Can you work these out from the model? Positions are in its coordinate system, mm. A direction names the side the tool comes from. Give positions to 0.01 mm unless a question says otherwise; leave off trailing zeros. Order: outer loops, then holes, each group sorted by start corner. A loop starts at its lowest first (then second) coordinate and runs counter-clockwise, first axis right, second up. Notation, with made-up numbers: (12, 44.5) - (39, 44.5) arc R19 cw to (39, 61.5) - close; hole circle Ø2 at (-0.5, 67). An arc over 180 degrees is marked (long way). Answer as a JSON object with one key per item and string values.
```python
from build123d import *

# Parameters (mm, degrees)
EXTRUDE_2_DEPTH = 5


with BuildPart() as part:
    # 草图1 → 凸台-拉伸2 (new body)
    with BuildSketch(Plane(origin=(0, 0, 0), x_dir=(1, 0, 0), z_dir=(0, 1, 0))):
        with BuildLine():
            Line((-5, 0), (7, 0))
            ThreePointArc((7, 0), (9.121320344, 0.878679656), (10, 3))
            Line((10, 3), (10, 6))
            ThreePointArc((10, 6), (10.878679656, 8.121320344), (13, 9))
            Line((13, 9), (177, 9))
            ThreePointArc((177, 9), (179.121320344, 8.121320344), (180, 6))
            Line((180, 6), (180, 3))
            ThreePointArc((180, 3), (180.878679656, 0.878679656), (183, 0))
            Line((183, 0), (195, 0))
            Line((195, 0), (195, 10))
            Line((195, 10), (190, 10))
            Line((190, 10), (190, 15))
            Line((190, 15), (170, 15))
            Line((170, 15), (170, 20))
            Line((170, 20), (160, 20))
            Line((160, 20), (160, 15))
            Line((160, 15), (105, 15))
            Line((105, 15), (105, 20))
            Line((105, 20), (85, 20))
            Line((85, 20), (85, 15))
            Line((85, 15), (30, 15))
            Line((30, 15), (30, 20))
            Line((30, 20), (20, 20))
            Line((20, 20), (20, 15))
            Line((20, 15), (0, 15))
            Line((0, 15), (0, 10))
            Line((0, 10), (-5, 10))
            Line((-5, 10), (-5, 15))
            Line((-5, 15), (-35, 15))
            Line((-35, 15), (-35, 10))
            Line((-35, 10), (-40, 10))
            Line((-40, 10), (-40, 0))
            Line((-40, 0), (-5, 0))
        make_face()
    extrude(amount=EXTRUDE_2_DEPTH)


solid = part.part
```
Q1. If we section it at C-C, the plane x = 124.5: Please give me the cut outline in (y, z), then the cut area to 3 significant figures.
Recorded:
{"outline": "(0, -15) - (5, -15) - (5, -9) - (0, -9) - close", "area": "30.0 mm^2"}
Q2. I need wall thicknesses on L1, parallel to X at y = 3.75, z = -15.5; L2, parallel to X at y = 1.3, z = -3.75; L3, parallel to X at y = 2.65, z = -14.75. Which ranges of each line are inside material? Lowest first, please.
Recorded:
{"L1": "x = 20 to 30, 85 to 105, 160 to 170", "L2": "x = -40 to 10, 180 to 195", "L3": "x = -35 to -5, 0 to 190"}
Q3. If we section it at A-A, the plane z = -17.75: Please give me the cut outline in (x, y), then the cut area to 3 significant figures.
Recorded:
{"outline": "(20, 0) - (30, 0) - (30, 5) - (20, 5) - close; (85, 0) - (105, 0) - (105, 5) - (85, 5) - close; (160, 0) - (170, 0) - (170, 5) - (160, 5) - close", "area": "200 mm^2"}
Q4. I'm going to push flat-ended pins straight in: pin 1 Ø1.5 at (x, y) = (175, 3.5) entering from -Z; pin 2 Ø2.5 at (y, z) = (2, -17) entering from -X; pin 3 Ø1.5 at (x, y) = (40.5, 2) entering from +Z; pin 4 Ø5 at (x, z) = (103.5, -5.5) entering from +Y. Where does each tip first touch, or does it pass through?
Recorded:
{"pin 1": "stops at z = -15", "pin 2": "stops at x = 20", "pin 3": "stops at z = -9", "pin 4": "passes through"}
Q5. Which directions (+Z, -Z, +X, -X, +Y, -Y) give clear straight access to the entire face, cutting with the end or side of a thin tool? Please do faces 1 (the face through (85, 2, -18)), 2 (the face through (189, 2, 0)), 3 (the face through (-20, 2, -15)), 4 (the face through (170, 2, -17)).
Recorded:
{"face 1": "-Z, +Y, -Y", "face 2": "+Z, +X, -X, +Y, -Y", "face 3": "-Z, -X, +Y, -Y", "face 4": "-Z, +X, +Y, -Y"}
Q6. We'd pull the mould along X, two halves only. Please class faces 5 (the face through (190, 2, -12)), 6 (the face through (25, 2, -20)), 7 (the face through (94, 2, -9)): released by +X, released by -X, zero draft, split by the parting line, or undercut.
Recorded:
{"face 5": "released by +X", "face 6": "zero draft", "face 7": "undercut"}
